from build123d import *

# Parameters (mm, degrees)
F1_R     = 10
F3_DEPTH = 0.5
F2_R     = 5.5
F4_DEPTH = 25
F9_DEPTH = 0.5


with BuildPart() as f3:
    # F1 (on Front) → F3 (new body)
    with BuildSketch(Plane.XZ):
        Circle(F1_R)
    extrude(amount=F3_DEPTH)

    # F2 (on Front) → F4 (cut)
    with BuildSketch(Plane.XZ):
        Circle(F2_R)
    extrude(amount=F4_DEPTH, mode=Mode.SUBTRACT)



with BuildPart() as f5_1:
    # F5: copy of F3
    add(f3.part.moved(Location((35, 0, 0))))


with BuildPart() as f6_1:
    # F6: copy of F3
    add(f3.part.moved(Location((105, 0, 0))))


with BuildPart() as f7_1:
    # F7: copy of F3
    add(f3.part.moved(Location((70, 0, 0))))


with BuildPart() as f3_1:
    add(f3.part)

    add(f5_1.part)  # F9 merges F5_1

    add(f6_1.part)  # F9 merges F6_1

    add(f7_1.part)  # F9 merges F7_1
    # F8 (on Front) → F9 (join)
    with BuildSketch(Plane.XZ):
        with BuildLine():
            ThreePointArc((28.654308, 7.728661), (17.5, 3.336749), (6.345692, 7.728661))
            Line((6.345692, 7.728661), (6.345692, -7.728661))
            ThreePointArc((6.345692, -7.728661), (17.5, -3.336749), (28.654308, -7.728661))
            Line((28.654308, -7.728661), (28.654308, 7.728661))
        make_face()
        with BuildLine():
            ThreePointArc((63.654308, 7.728661), (52.5, 3.336749), (41.345692, 7.728661))
            Line((41.345692, 7.728661), (41.345692, -7.728661))
            ThreePointArc((41.345692, -7.728661), (52.5, -3.336749), (63.654308, -7.728661))
            Line((63.654308, -7.728661), (63.654308, 7.728661))
        make_face()
        with BuildLine():
            ThreePointArc((98.654308, 7.728661), (87.5, 3.336749), (76.345692, 7.728661))
            Line((76.345692, 7.728661), (76.345692, -7.728661))
            ThreePointArc((76.345692, -7.728661), (87.5, -3.336749), (98.654308, -7.728661))
            Line((98.654308, -7.728661), (98.654308, 7.728661))
        make_face()
    extrude(amount=F9_DEPTH)


solid = f3_1.part
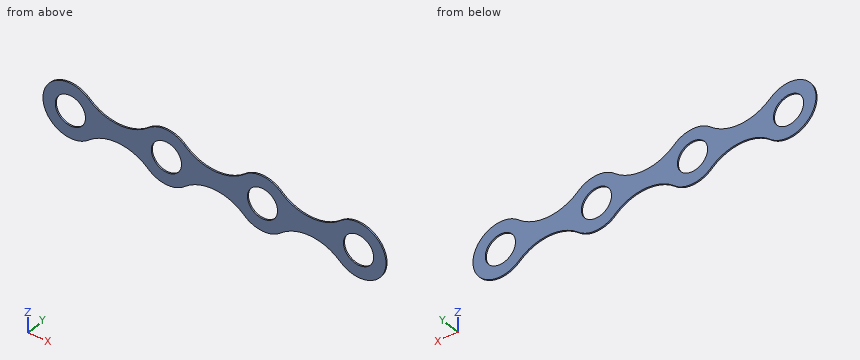
Here's how the part is built. I have some questions about the finished solid (model axes, mm). Coordinates: 2 decimals unless noted, no trailing zeros. Write each loop counter-clockwise with the first axis right and the second up, starting at its lowest first coordinate (ties: lowest second). Pieces come first, ordered by that corner, then holes.
1) If we section it at C-C (z = -1.25): List the corners of the cut face in (x, y) for me.
Filled in:
outline: (-9.92, -0.5) - (-5.36, -0.5) - (-5.36, 0) - (-9.92, 0) - close; (5.36, -0.5) - (29.64, -0.5) - (29.64, 0) - (5.36, 0) - close; (40.36, -0.5) - (64.64, -0.5) - (64.64, 0) - (40.36, 0) - close; (75.36, -0.5) - (99.64, -0.5) - (99.64, 0) - (75.36, 0) - close; (110.36, -0.5) - (114.92, -0.5) - (114.92, 0) - (110.36, 0) - close
2) If I drill on line 1 (X direction, y = -0.1, z = 0); line 2 (Z direction, x = 105, y = -0.3); line 3 (X direction, y = -0.1, z = 6.75), over which ranges is the centre line in solid material (lowest first)?
Filled in:
line 1: x = -10 to -5.5, 5.5 to 29.5, 40.5 to 64.5, 75.5 to 99.5, 110.5 to 115
line 2: z = -10 to -5.5, 5.5 to 10
line 3: x = -7.38 to 7.5, 27.5 to 42.5, 62.5 to 77.5, 97.5 to 112.38
3) If we section it at A-A (x = 35): List the corners of the cut face in (y, z) for me, plus the area to 3 significant figures.
Filled in:
outline: (-0.5, -10) - (0, -10) - (0, -5.5) - (-0.5, -5.5) - close; (-0.5, 5.5) - (0, 5.5) - (0, 10) - (-0.5, 10) - close
area: 4.50 mm2
4) If we section it at B-B (y = -0.4): List the corners of the cut face in (x, z) for me, plus the area to 3 significant figures.
Filled in:
outline: (6.93, -7.21) arc R16.36 cw to (28.07, -7.21) arc R10 ccw to (41.93, -7.21) arc R16.36 cw to (63.07, -7.21) arc R10 ccw to (76.93, -7.21) arc R16.36 cw to (98.07, -7.21) arc R10 ccw (long way) to (98.07, 7.21) arc R16.36 cw to (76.93, 7.21) arc R10 ccw to (63.07, 7.21) arc R16.36 cw to (41.93, 7.21) arc R10 ccw to (28.07, 7.21) arc R16.36 cw to (6.93, 7.21) arc R10 ccw (long way) to start; hole circle Ø11 at (0, 0); hole circle Ø11 at (35, 0); hole circle Ø11 at (70, 0); hole circle Ø11 at (105, 0)
area: 1,270 mm2
5) I'm going to push a flat-ended pin straight in: pin 1 (6.5 mm diameter, centred on x = 35, z = 0, fed in from -Y). Where does the tip first touch, or does it pass through?
Filled in:
pin 1: passes through
6) If we section it at D-D (x = 106): List the corners of the cut face in (y, z) for me.
Filled in:
outline: (-0.5, -9.95) - (0, -9.95) - (0, -5.41) - (-0.5, -5.41) - close; (-0.5, 5.41) - (0, 5.41) - (0, 9.95) - (-0.5, 9.95) - close
